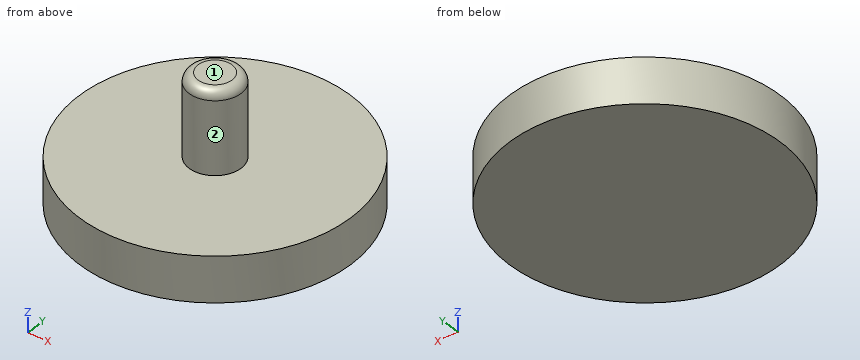
from build123d import *

# Parameters (mm, degrees)
SKETCH1_R           = 7.5
BOSS_EXTRUDE1_DEPTH = 2.5
SKETCH2_R           = 1.4375
BOSS_EXTRUDE2_DEPTH = 4.5
FILLET1_R           = 0.5


with BuildPart() as part:
    # Sketch1 → Boss-Extrude1 (new body)
    with BuildSketch(Plane.XY):
        Circle(SKETCH1_R)
    extrude(amount=BOSS_EXTRUDE1_DEPTH)

    # Sketch2 → Boss-Extrude2 (add)
    with BuildSketch(Plane.XY.offset(2.5)):
        Circle(SKETCH2_R)
    extrude(amount=BOSS_EXTRUDE2_DEPTH)

    # Fillet1
    fillet1_edges = [part.edges().sort_by_distance(p)[0] for p in [
        (-1.4375, 0, 7),
    ]]
    fillet(fillet1_edges, radius=FILLET1_R)


solid = part.part
Source: CAD feature listing. Evaluate the final solid. Frame: model axes, mm. Face numbers are marked on the shaded views. A direction names the side the tool comes from. Give positions to 0.01 mm unless a question says otherwise; leave off trailing zeros. Write each loop counter-clockwise with the first axis right and the second up, starting at its lowest first coordinate (ties: lowest second). Pieces come first, ordered by that corner, then holes. Notation, with made-up numbers: M 79,38.5 L 91,38.5 A19 cw 91,53.5 Z; hole C 68.5,78.5 d5. An arc over 180 degrees is marked long. Answer as a JSON object with one key per item and string values.
Q1. Access query for the marked faces 1 and 2. Directions: +Z, -Z, +X, -X, +Y, -Y. A direction counts if a zero-diameter tool reaches every point of the face in a straight line with its end or side. Return the directions, or none.
Geometry check:
{"face 1": "+Z, +X, -X, +Y, -Y", "face 2": "+Z"}
Q2. Contact query for flat-ended pins moving along their axis: P1, Ø2, axis at x = 0.5, z = 3, coming from the +Y side; P2, Ø2, axis at x = 5.5, z = 2.5, coming from the +Y side. Output: stop coordinate, or through.
Geometry check:
{"P1": "stops at y = 7.5", "P2": "stops at y = 6"}
Q3. Ray query, line 1 along Z through (x, y) = (1.5, 3); line 2 along Y through (x, z) = (-4.25, 1.25); line 3 along X through (y, z) = (5, 2.25). Return the intervals inside material, ascending.
Geometry check:
{"line 1": "z = 0 to 2.5", "line 2": "y = -6.18 to 6.18", "line 3": "x = -5.59 to 5.59"}
Q4. Cut plane C-C, the plane z = 6. Return the cut outline in (x, y) (1 decimal).
Geometry check:
{"outline": "C 0,0 d2.9"}
Q5. Cut plane A-A, the plane y = 0. Return the cut outline in (x, z), then the cut area to 3 significant figures.
Geometry check:
{"outline": "M -7.5,0 L 7.5,0 L 7.5,2.5 L 1.44,2.5 L 1.44,6.5 A0.5 ccw 0.94,7 L -0.94,7 A0.5 ccw -1.44,6.5 L -1.44,2.5 L -7.5,2.5 Z", "area": "50.3 mm^2"}
Q6. Cut plane D-D, the plane z = 0.5. Return the cut outline in (x, y), then the cut area to 3 significant figures.
Geometry check:
{"outline": "C 0,0 d15", "area": "177 mm^2"}
